Part model, mm, in its own coordinate system. A direction names the side the tool comes from. Coordinates: 2 decimals unless noted, no trailing zeros. Loops run counter-clockwise (first coordinate to the right, second up) from the corner with the lowest first, then second, coordinate; pieces in that order, holes last. Notation, with made-up numbers: M 15.5,46 L 47.5,46 A24 cw 47.5,57 Z; hole C 28,-34.75 d9. An arc over 180 degrees is marked long. Use a Markdown table: item, result. Add a question column.
1) Band-saw the part on D-D (x = -10.25). List the corners of the cut face in (y, z), plus the area to 3 significant figures.
2) Pin check, flat tips, straight feed: pin 1 Ø8 at (x, y) = (11, -13.5) entering from -Z; pin 2 Ø6 at (x, z) = (-5.45, 4.66) entering from -Y; pin 3 Ø5 at (y, z) = (-16, 2) entering from +X. Stop position of each tip, or through.
3) Band-saw the part on A-A (y = -2.5). List the corners of the cut face in (x, z).
4) Tool access for faces 1 (the flat face through (0, -10, -7.001)), 2 (the cylindrical face through (4.939, -17.535, 8.595)), 3 (the flat face through (-10.44, -9.86, -5.92)): list every direction of +Z, -Z, +X, -X, +Y, -Y with a clear straight run to the whole face (end or side of a thin tool).
5) Pull direction X, two halves, no side cores. Call faces 4 (the flat face through (-6, -15, 5)), 5 (the flat face through (0, -10, 12.001)), 6 (the cylindrical face through (-0.529, -13.705, -9.536)), 7 (the flat face through (-10.345, -9.86, 6.084)): released by +X, released by -X, zero draft, split by the parting line, or undercut.
6) Band-saw the part on B-B (z = -7.5). List the corners of the cut face in (x, y), plus the area to 3 significant figures.
7) Wall check: probe 1 along Y at (x, z) = (0, -9.2); probe 2 along X at (y, z) = (-17.5, 6); probe 3 along Z at (x, y) = (5.25, -16.75). Give the ranges that are in metal, low to high. Write a range as from..to.
8) Band-saw the part on C-C (z = 6.5). List the corners of the cut face in (x, y), plus the area to 3 significant figures.
from build123d import *

# Parameters (mm, degrees)
F1_DEPTH = 20
F2_R     = 3.9672544226
F2_R_2   = 3.7268973953
F4_DEPTH = 5
F6_R     = 4.0640636786
F7_DEPTH = 5
F8_DEPTH = 5


# Not quite as in the source:
# - the program builds the solid bodies; features that only make, move or delete a surface that nothing else refers to are left out


with BuildPart() as f1:
    # F0 (on Front) → F1 (new body)
    with BuildSketch(Plane.XZ):
        Polygon((-6.9287490553, -12.0009453967), (6.9287490553, -12.0009453967), (13.8574981107, 0), (6.9287490553, 12.0009453967), (-6.9287490553, 12.0009453967), (-13.8574981107, 0), align=None)
    extrude(amount=F1_DEPTH)

    # F2 (on face) → F4 (cut)
    with BuildSketch(Plane.XZ.offset(20)):
        with Locations((5.454974249, 4.6615242027)):
            Circle(F2_R)
        with Locations((-5.4549747147, 4.6615242027)):
            Circle(F2_R_2)
    extrude(amount=-F4_DEPTH, mode=Mode.SUBTRACT)

    # F6 (on face) → F7 (cut)
    with BuildSketch(Plane(origin=(0, 0, -12.0009453967), x_dir=(1, 0, 0), z_dir=(0, 0, -1))):
        with Locations((0, 9.6756508574)):
            Circle(F6_R)
    extrude(amount=-F7_DEPTH, mode=Mode.SUBTRACT)

    # F3 (on face) → F8 (cut)
    with BuildSketch(Plane.XZ.offset(20)):
        with BuildLine():
            Line((0, -5.3527420043), (0, -7.04187667))
            add(Edge.make_bspline(
                [(6.6451518796, -5.4549751803), (6.6575654316, -6.1571957747), (3.2728013866, -7.1077153996), (0, -7.04187667)],
                knots=[0.7456529131, 0.7456529131, 0.7456529131, 0.7456529131, 1, 1, 1, 1], degree=3))
            Line((6.6451518796, -5.4549751803), (0, -5.3527420043))
        make_face()
        with BuildLine():
            Line((0, -5.3527420043), (6.6451518796, -5.4549751803))
            add(Edge.make_bspline(
                [(0, -4.2647989467), (3.2636275259, -4.3042470372), (6.6328122368, -4.7569355417), (6.6451518796, -5.4549751803)],
                knots=[0.492820185, 0.492820185, 0.492820185, 0.492820185, 0.7456529131, 0.7456529131, 0.7456529131, 0.7456529131], degree=3))
            Line((0, -4.2647989467), (0, -5.3527420043))
        make_face()
        with BuildLine():
            add(Edge.make_bspline(
                [(-6.2484252267, -5.2566123195), (-6.2199094707, -4.57569338), (-3.1594165925, -4.2266104736), (0, -4.2647989467)],
                knots=[0.2480606621, 0.2480606621, 0.2480606621, 0.2480606621, 0.492820185, 0.492820185, 0.492820185, 0.492820185], degree=3))
            Line((-6.2484252267, -5.2566123195), (0, -5.3527420043))
            Line((0, -5.3527420043), (0, -4.2647989467))
        make_face()
        with BuildLine():
            add(Edge.make_bspline(
                [(0, -7.04187667), (-3.191911057, -6.9776652057), (-6.2773255825, -5.9467150004), (-6.2484252267, -5.2566123195)],
                knots=[0, 0, 0, 0, 0.2480606621, 0.2480606621, 0.2480606621, 0.2480606621], degree=3))
            Line((0, -7.04187667), (0, -5.3527420043))
            Line((0, -5.3527420043), (-6.2484252267, -5.2566123195))
        make_face()
    extrude(amount=-F8_DEPTH, mode=Mode.SUBTRACT)


solid = f1.part
Entries:
| question | item | result |
|---|---|---|
| 1 | outline | M -20,-6.25 L 0,-6.25 L 0,6.25 L -20,6.25 Z |
| 1 | area | 250 mm2 |
| 2 | pin 1 | z = -11.88 |
| 2 | pin 2 | y = -15 |
| 2 | pin 3 | x = 13.86 |
| 3 | outline | M -13.86,0 L -6.93,-12 L 6.93,-12 L 13.86,0 L 6.93,12 L -6.93,12 Z |
| 4 | face 1 | -Z |
| 4 | face 2 | -Y |
| 4 | face 3 | -Z, -X, +Y, -Y |
| 5 | face 4 | undercut |
| 5 | face 5 | zero draft |
| 5 | face 6 | undercut |
| 5 | face 7 | released by -X |
| 6 | outline | M -9.53,-20 L 9.53,-20 L 9.53,0 L -9.53,0 Z; hole C 0,-9.68 d8.13 |
| 6 | area | 329 mm2 |
| 7 | probe 1 | -20..-13.74, -5.61..0 |
| 7 | probe 2 | -10.39..-8.93, -1.98..1.72, 9.19..10.39 |
| 7 | probe 3 | -12..-6.34, -4.75..0.7, 8.62..12 |
| 8 | outline | M -10.1,-20 L -8.7,-20 L -8.7,-15 L -2.21,-15 L -2.21,-20 L 1.94,-20 L 1.94,-15 L 8.97,-15 L 8.97,-20 L 10.1,-20 L 10.1,0 L -10.1,0 Z |
| 8 | area | 337 mm2 |
